The listing builds one solid part. Answer for the finished solid, in the listing's coordinates (mm). Coordinates: 2 decimals unless noted, no trailing zeros. Write each loop counter-clockwise with the first axis right and the second up, starting at its lowest first coordinate (ties: lowest second). Pieces come first, ordered by that corner, then holes.
(1) Straight lines are drawn through the part: line 1 (X direction, y = -14.25, z = 29); line 2 (Z direction, x = -565.5, y = -9); line 3 (X direction, y = -11.5, z = -49.5). For each, find the intervals that lie inside material, in ascending order.
(2) Given P1, Ø7, axis at y = -9, z = -45, coming from the +X side; P2, Ø6, axis at x = 15, y = -5.5, coming from the -Z side; P3, Ø7, axis at x = -349, z = -45, coming from the -Y side, each flat-ended and moving along its own axis, determine where each tip first touches the part or whether it passes through.
(3) The part is cut by section A-A on x = 25. Determine the outline of the cut face in (y, z).
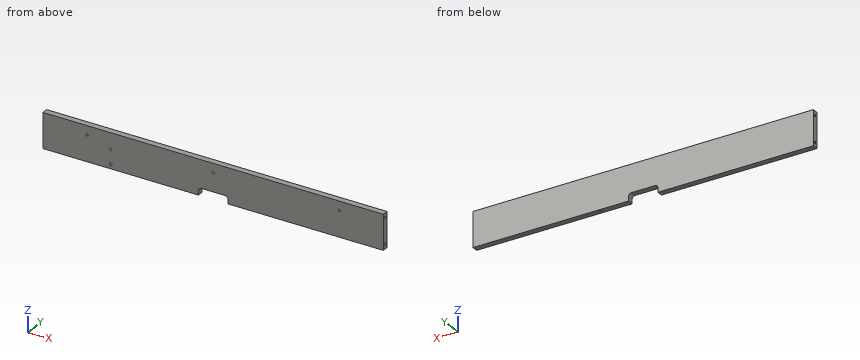
from build123d import *

# Parameters (mm, degrees)
F0_W           = 1160
F0_H           = 120
F1_DEPTH       = 20
F3_DEPTH       = 20.001
F8_D           = 8
F8_DEPTH       = 30
F8_TIP         = 2.4034424761
F8_ON_F5_D     = 8
F8_ON_F5_DEPTH = 30
F8_ON_F5_TIP   = 2.4034424761
F8_ON_F7_D     = 8
F8_ON_F7_DEPTH = 30
F8_ON_F7_TIP   = 2.4034424761
F9_D           = 8
F9_DEPTH       = 10
F9_TIP         = 2.4034424761


with BuildPart() as f1:
    # F0 (on Front) → F1 (new body)
    with BuildSketch(Plane.XZ):
        Rectangle(F0_W, F0_H)
    extrude(amount=F1_DEPTH)

    # F2 (on face) → F3 (cut, through all)
    with BuildSketch(Plane.XZ.offset(20)):
        with BuildLine():
            Line((-50, -45), (-50, -60))
            Line((-50, -60), (50, -60))
            Line((50, -60), (50, -45))
            ThreePointArc((50, -45), (47.0710678119, -37.9289321881), (40, -35))
            Line((40, -35), (-40, -35))
            ThreePointArc((-40, -35), (-47.0710678119, -37.9289321881), (-50, -45))
        make_face()
    extrude(amount=-F3_DEPTH, mode=Mode.SUBTRACT)

    # F8
    with Locations(Plane(origin=(-580, 0, 0), x_dir=(0, -1, 0), z_dir=(-1, 0, 0))):
        with Locations((9, 45), (9, -45)):
            Hole(F8_D / 2, depth=F8_DEPTH)
            with Locations((0, 0, -(F8_DEPTH + F8_TIP / 2))):  # 118° drill point
                Cone(0, F8_D / 2, F8_TIP, mode=Mode.SUBTRACT)

    # F8 on F5
    with Locations(Plane.YZ.offset(580)):
        with Locations((-9, 45), (-9, -45)):
            Hole(F8_ON_F5_D / 2, depth=F8_ON_F5_DEPTH)
            with Locations((0, 0, -(F8_ON_F5_DEPTH + F8_ON_F5_TIP / 2))):  # 118° drill point
                Cone(0, F8_ON_F5_D / 2, F8_ON_F5_TIP, mode=Mode.SUBTRACT)

    # F8 on F7
    with Locations(Plane(origin=(0, 0, -60), x_dir=(1, 0, 0), z_dir=(0, 0, -1))):
        with Locations((-430, 9), (-150, 9), (150, 9), (430, 9)):
            Hole(F8_ON_F7_D / 2, depth=F8_ON_F7_DEPTH)
            with Locations((0, 0, -(F8_ON_F7_DEPTH + F8_ON_F7_TIP / 2))):  # 118° drill point
                Cone(0, F8_ON_F7_D / 2, F8_ON_F7_TIP, mode=Mode.SUBTRACT)

    # F9
    with Locations(Plane.XZ.offset(20)):
        with Locations((430, 29), (0, 29), (-430, 29), (-349, -45), (-349, 5)):
            Hole(F9_D / 2, depth=F9_DEPTH)
            with Locations((0, 0, -(F9_DEPTH + F9_TIP / 2))):  # 118° drill point
                Cone(0, F9_D / 2, F9_TIP, mode=Mode.SUBTRACT)


solid = f1.part
Model answer:
1. line 1: x = -580 to -434, -426 to -4, 4 to 426, 434 to 580
1. line 2: z = -60 to -49, -41 to 41, 49 to 60
1. line 3: x = -580 to -433.12, -426.88 to -153.12, -146.88 to -50, 50 to 146.88, 153.12 to 426.88, 433.12 to 580
2. P1: stops at x = 549.7
2. P2: stops at z = -35
2. P3: stops at y = -9.7
3. outline: (-20, -35) - (0, -35) - (0, 60) - (-20, 60) - close
